from build123d import *

# Parameters (mm, degrees)
SKETCH_1_W          = 80
SKETCH_1_H          = 22
EXTRUDE_1_DEPTH     = 1.6
SKETCH_2_W          = 13
SKETCH_2_H          = 13
EXTRUDE_2_DEPTH     = 3.5
SKETCH_4_R          = 7
EXTRUDE_3_DEPTH     = 14
SKETCH_5_R          = 1.1
CUT_EXTRUDE_1_DEPTH = 2.6
EXTRUDE_4_DEPTH     = 2.8


with BuildPart() as part:
    # 草图1 → 凸台-拉伸1 (new body)
    with BuildSketch(Plane(origin=(0, 0, 0), x_dir=(1, 0, 0), z_dir=(0, 1, 0))):
        Rectangle(SKETCH_1_W, SKETCH_1_H)
    extrude(amount=EXTRUDE_1_DEPTH)

    # 草图2 → 凸台-拉伸2 (add)
    with BuildSketch(Plane(origin=(0, 1.6, 0), x_dir=(1, 0, 0), z_dir=(0, 1, 0))):
        with Locations((30.5, 0)):
            Rectangle(SKETCH_2_W, SKETCH_2_H)
        with Locations((-30.5, 0)):
            Rectangle(SKETCH_2_W, SKETCH_2_H)
    extrude(amount=EXTRUDE_2_DEPTH)

    # 草图4 → 凸台-拉伸3 (add)
    with BuildSketch(Plane(origin=(0, 5.1, 0), x_dir=(1, 0, 0), z_dir=(0, 1, 0))):
        with Locations((-30.65, 0)):
            Circle(SKETCH_4_R)
        with Locations((30.65, 0)):
            Circle(SKETCH_4_R)
    extrude(amount=EXTRUDE_3_DEPTH)

    # 草图5 → 切除-拉伸1 (cut, through all)
    with BuildSketch(Plane(origin=(0, 1.6, 0), x_dir=(1, 0, 0), z_dir=(0, 1, 0))):
        with Locations((-38.1, 9.1)):
            Circle(SKETCH_5_R)
        with Locations((-38.1, -9.1)):
            Circle(SKETCH_5_R)
        with Locations((38.1, -9.1)):
            Circle(SKETCH_5_R)
        with Locations((38.1, 9.1)):
            Circle(SKETCH_5_R)
    extrude(amount=-CUT_EXTRUDE_1_DEPTH, mode=Mode.SUBTRACT)

    # 草图6 → 凸台-拉伸4 (add)
    with BuildSketch(Plane(origin=(0, 1.6, 0), x_dir=(1, 0, 0), z_dir=(0, 1, 0))):
        Polygon((0, -11), (-2, -11), (-2, -5.136292724), (2, -5.136292724), (2, -11), align=None)
    extrude(amount=EXTRUDE_4_DEPTH)


solid = part.part
Work out the finished part from the listing and answer in its coordinate system (mm). A direction names the side the tool comes from. Coordinates: 2 decimals unless noted, no trailing zeros. Write each loop counter-clockwise with the first axis right and the second up, starting at its lowest first coordinate (ties: lowest second). Pieces come first, ordered by that corner, then holes.
1. The part is cut by section A-A, the plane z = 9.1. Write down the section's boundary in (x, y), and give its area (3 significant figures).
Results list:
outline: (-40, 0) - (-39.2, 0) - (-39.2, 1.6) - (-40, 1.6) - close; (-37, 0) - (37, 0) - (37, 1.6) - (2, 1.6) - (2, 4.4) - (-2, 4.4) - (-2, 1.6) - (-37, 1.6) - close; (39.2, 0) - (40, 0) - (40, 1.6) - (39.2, 1.6) - close
area: 132 mm2
2. For a pull along Y with two mould halves and no side action, classify faces 4 (the flat face through (-31, 19.1, 0)), 5 (the flat face through (30, 3, 6.5)), 6 (the cylindrical face through (-37.643, 12.002, -0.308)) as +Y half, -Y half, draft (parallel to the pull), parting line (faces both ways), or undercut.
Results list:
face 4: +Y half
face 5: undercut
face 6: draft
3. The part is cut by section B-B, the plane y = 3. Write down the section's boundary in (x, z), and give its area (3 significant figures).
Results list:
outline: (-37, -6.5) - (-24, -6.5) - (-24, 6.5) - (-37, 6.5) - close; (-2, 5.14) - (2, 5.14) - (2, 11) - (-2, 11) - close; (24, -6.5) - (37, -6.5) - (37, 6.5) - (24, 6.5) - close
area: 361 mm2
4. The part is cut by section D-D, the plane x = 30.65. Write down the section's boundary in (y, z), and give its area (3 significant figures).
Results list:
outline: (0, -11) - (1.6, -11) - (1.6, -6.5) - (5.1, -6.5) - (5.1, -7) - (19.1, -7) - (19.1, 7) - (5.1, 7) - (5.1, 6.5) - (1.6, 6.5) - (1.6, 11) - (0, 11) - close
area: 277 mm2
5. For faces 1 (the flat face through (-2, 3, 8)), 2 (the flat face through (30, 3, -6.5)), 3 (the flat face through (25, 5.1, -5)), determine the directions among +Z, -Z, +X, -X, +Y, -Y from which every point of the face is accessible in a straight line to the end or side of a thin tool.
Results list:
face 1: +Z, -Z, +Y
face 2: -Z, +X, -X
face 3: -Z, +Y
6. The part is cut by section C-C, the plane z = 0. Write down the section's boundary in (x, y), and give its area (3 significant figures).
Results list:
outline: (-40, 0) - (40, 0) - (40, 1.6) - (37, 1.6) - (37, 5.1) - (37.65, 5.1) - (37.65, 19.1) - (23.65, 19.1) - (23.65, 5.1) - (24, 5.1) - (24, 1.6) - (-24, 1.6) - (-24, 5.1) - (-23.65, 5.1) - (-23.65, 19.1) - (-37.65, 19.1) - (-37.65, 5.1) - (-37, 5.1) - (-37, 1.6) - (-40, 1.6) - close
area: 611 mm2
7. Consider line 1 along X through (y, z) = (0.65, 9.1); line 2 along Z through (x, y) = (-38.1, 1); line 3 along X through (y, z) = (3, -6.25). Determine where each line is inside the solid, lowest interval first.
Results list:
line 1: x = -40 to -39.2, -37 to 37, 39.2 to 40
line 2: z = -11 to -10.2, -8 to 8, 10.2 to 11
line 3: x = -37 to -24, 24 to 37
8. Flat-ended cylindrical pins translate along their axes: pin 1 (1.8 mm diameter, centred on x = 38.1, z = -9.1, fed in from -Y) (1 decimal); pin 2 (3 mm diameter, centred on y = 12.5, z = -5.5, fed in from +X); pin 3 (1.5 mm diameter, centred on y = 2.5, z = -1, fed in from -X); pin 4 (2 mm diameter, centred on y = 16, z = 5, fed in from -X). Find the tip coordinate at first contact, or state that the pin passes through.
Results list:
pin 1: passes through
pin 2: stops at x = 36.39
pin 3: stops at x = -37
pin 4: stops at x = -36.39
